from build123d import *

# Parameters (mm, degrees)
M3_CLEARANCE_HOLE1_D     = 3.4
M3_CLEARANCE_HOLE1_DEPTH = 4
M3_CLEARANCE_HOLE1_TIP   = 1.021463052
SKETCH5_R                = 29.5
CUT_EXTRUDE1_DEPTH       = 1


with BuildPart() as part:
    # Sketch1 → Revolve1 (revolve)
    with BuildSketch(Plane.XY, mode=Mode.PRIVATE) as revolve1_sk:
        Polygon((0, -7.4), (0, 7.4), (-28, 7.4), (-31.5, 4.9), (-31.5, -7.4), align=None)
    revolve(revolve1_sk.sketch.rotate(Axis((0, -7.4, 0), (0, 1, 0)), 180), axis=Axis((0, -7.4, 0), (0, 1, 0)))

    # M3 Clearance Hole1
    with Locations(Plane(origin=(0, 7.4, 0), x_dir=(1, 0, 0), z_dir=(0, 1, 0))):
        with Locations((-15.556349186, 15.556349186), (-10.606601718, 10.606601718), (0, 12.5), (10.606601718, 10.606601718), (15.556349186, 15.556349186), (0, -12.5), (-12.5, 0), (12.5, 0), (10.606601718, -10.606601718), (-10.606601718, -10.606601718), (-15.556349186, -15.556349186), (15.556349186, -15.556349186)):
            Hole(M3_CLEARANCE_HOLE1_D / 2, depth=M3_CLEARANCE_HOLE1_DEPTH)
            with Locations((0, 0, -(M3_CLEARANCE_HOLE1_DEPTH + M3_CLEARANCE_HOLE1_TIP / 2))):  # 118° drill point
                Cone(0, M3_CLEARANCE_HOLE1_D / 2, M3_CLEARANCE_HOLE1_TIP, mode=Mode.SUBTRACT)

    # Sketch5 → Cut-Extrude1 (cut)
    with BuildSketch(Plane.XZ.offset(7.4)):
        Circle(SKETCH5_R)
    extrude(amount=-CUT_EXTRUDE1_DEPTH, mode=Mode.SUBTRACT)


solid = part.part
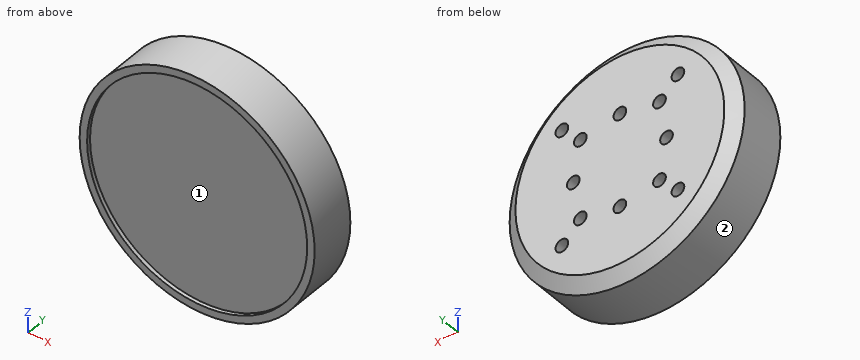
Geometry: final body of the model. Coordinates: model frame, mm. Face numbers are marked on the shaded views. A direction names the side the tool comes from. Give positions to 0.01 mm unless a question says otherwise; leave off trailing zeros. Order: outer loops, then holes, each group sorted by start corner. A loop starts at its lowest first (then second) coordinate and runs counter-clockwise, first axis right, second up. Notation, with made-up numbers: (0.5, 28) -> (47.5, 28) arc R14 ccw to (47.5, 45) -> close; hole circle Ø1 at (66.25, 46). An arc over 180 degrees is marked (long way). Write each question's results on one line, items separated by ' | '.
1) Cut plane A-A (y = -3). Output: boundary loops of the cut face in (x, z), and give its area (3 significant figures).
Geometry says:
outline: circle Ø63 at (0, 0) | area: 3,120 mm²
2) Line query: line 1 along X through (y, z) = (5, -0.5); line 2 along Y through (x, z) = (-15, -18.5); line 3 along Z through (x, y) = (-12.5, 6.05). Output: solid intervals per line, ascending.
Geometry says:
line 1: x = -31.36 to -14.12, -10.88 to 10.88, 14.12 to 31.36 | line 2: y = -6.4 to 7.4 | line 3: z = -27.15 to -1.7, 1.7 to 27.15
3) Set-up query: the marked faces 1 and 2. Return all of +Z, -Z, +X, -X, +Y, -Y with unobstructed straight access to the full face (end or side cutting, diameter ignored); none if empty.
Geometry says:
face 1: -Y | face 2: +Y, -Y
4) First-contact query: pin 1 Ø3 at (x, y) = (-4, 0.5) entering from +Z; pin 2 Ø2 at (x, z) = (15.56, -15.56) entering from -Y; pin 3 Ø1 at (x, y) = (6.5, 4) entering from +Z. Flat tips, straight axial feed; report the tip coordinate or a pass-through.
Geometry says:
pin 1: stops at z = 31.4 | pin 2: stops at y = -6.4 | pin 3: stops at z = 30.92
